```python
from build123d import *
from build123d.topology import SkipClean

# Parameters (mm, degrees)
SKETCH1_R               = 15
SKETCH1_R_2             = 12.5
BOSS_EXTRUDE2_DEPTH     = 2.5
CUT_EXTRUDE2_DEPTH      = 22.360009363
CUT_EXTRUDE2_DEPTH_BACK = 22.360009363
SKETCH3_R               = 0.45
SKETCH4_R               = 1.25
BOSS_EXTRUDE3_DEPTH     = 18
BOSS_EXTRUDE4_START     = -20
SKETCH6_R               = 1.25
BOSS_EXTRUDE4_DEPTH     = 20
SKETCH9_R               = 1.75
BOSS_EXTRUDE5_DEPTH     = 2


with BuildPart() as part:
    # Sketch1 → Boss-Extrude2 (new body)
    with BuildSketch(Plane(origin=(0, 0, 0), x_dir=(1, 0, 0), z_dir=(0, 1, 0))):
        with Locations(Location((0, 0, 0), (0, 0, 270))):
            Circle(SKETCH1_R)
        with Locations(Location((0, 0, 0), (0, 0, 270))):
            Circle(SKETCH1_R_2, mode=Mode.SUBTRACT)
    extrude(amount=BOSS_EXTRUDE2_DEPTH)

    # Sketch3 → Cut-Extrude2 (cut, two sides: drawn at the far end of the back side and taken through both)
    with BuildSketch(Plane.XY.offset(-CUT_EXTRUDE2_DEPTH_BACK)):
        with Locations(Location((0, 1.25, 0), (0, 0, 89.999999951))):
            Circle(SKETCH3_R)
    extrude(amount=CUT_EXTRUDE2_DEPTH + CUT_EXTRUDE2_DEPTH_BACK, mode=Mode.SUBTRACT)

    # Sketch4 → Boss-Extrude3 (add)
    with SkipClean():  # the faces are left unmerged after this step: merging them gives an invalid solid
        with BuildSketch(Plane(origin=(14, 0, 0), x_dir=(0, 0, -1), z_dir=(1, 0, 0))):
            with Locations(Location((0, 1.25, 0), (0, 0, 90))):
                Circle(SKETCH4_R)
        extrude(amount=BOSS_EXTRUDE3_DEPTH)

    # Sketch5 → Revolve1 (revolve)
    with SkipClean():  # the faces are left unmerged after this step: merging them gives an invalid solid
        with BuildSketch(Plane(origin=(32, 0, 0), x_dir=(0, 0, -1), z_dir=(1, 0, 0))):
            with BuildLine():
                Line((0, 2.5), (0, 0))
                ThreePointArc((0, 0), (1.25, 1.25), (0, 2.5))
            make_face()
        revolve(axis=Axis((32, 2.5, 0), (0, -1, 0)))

    # Sketch6 → Boss-Extrude4 (add)
    with BuildSketch(Plane(origin=(-14, 0, 0), x_dir=(0, 0, -1), z_dir=(1, 0, 0)).offset(BOSS_EXTRUDE4_START)):
        with Locations(Location((0, 1.25, 0), (0, 0, 90))):
            Circle(SKETCH6_R)
    extrude(amount=BOSS_EXTRUDE4_DEPTH)

    # Sketch7 → Revolve2 (revolve)
    with BuildSketch(Plane.ZY.offset(34)):
        with BuildLine():
            Line((0, 2.5), (0, 0))
            ThreePointArc((0, 0), (1.25, 1.25), (0, 2.5))
        make_face()
    revolve(axis=Axis((-34, 2.5, 0), (0, -1, 0)))

    # Sketch9 → Boss-Extrude5 (add)
    with BuildSketch(Plane(origin=(24, 0, 0), x_dir=(0, 0, -1), z_dir=(1, 0, 0))):
        with Locations((0, 1.25)):
            Circle(SKETCH9_R)
    extrude(amount=-BOSS_EXTRUDE5_DEPTH)


solid = part.part
```
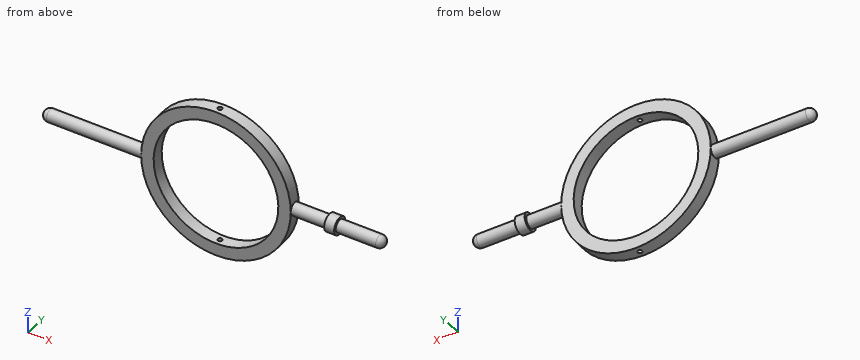
Part model, mm, in its own coordinate system. Round coordinates to 2 decimals unless told otherwise and drop trailing zeros. Loops run counter-clockwise (first coordinate to the right, second up) from the corner with the lowest first, then second, coordinate; pieces in that order, holes last. Notation, with made-up numbers: (-22, -32) -> (-16, -32) arc R26 cw to (-16, -15) -> close; hole circle Ø3 at (32.25, -34.75). An arc over 180 degrees is marked (long way). Use one line per item in the form item = value. Start each with the question number.
Item 1: Band-saw the part on B-B (z = 3). List the corners of the cut face in (x, y), plus the area to 3 significant figures.
Item 2: Band-saw the part on C-C (x = 28). List the corners of the cut face in (y, z).
Item 3: Drop flat-ended pins along their axis: pin 1 Ø1.5 at (y, z) = (0.5, 5.5) entering from -X; pin 2 Ø2 at (x, y) = (-17, 2) entering from +Z; pin 3 Ø1 at (y, z) = (0.5, -0.5) entering from -X. Give the stop position or say it passes through.
Item 4: Band-saw the part on A-A (x = -6.5). List the corners of the cut face in (y, z).
Item 5: Drill centre lines: line 1 along Z through (x, y) = (0, 0.6); line 2 along X through (y, z) = (0.3, -2); line 3 along X through (y, z) = (1.25, 13.55). Where is each one in solid material? Low to high.
Data:
q1.outline = (-14.7, 0) -> (-12.13, 0) -> (-12.13, 2.5) -> (-14.7, 2.5) -> close; (12.13, 0) -> (14.7, 0) -> (14.7, 2.5) -> (12.13, 2.5) -> close
q1.area = 12.8 mm^2
q2.outline = circle Ø2.5 at (1.25, 0)
q3.pin_1 = -14.23
q3.pin_2 = 1.25
q3.pin_3 = -35.18
q4.outline = (0, -13.52) -> (2.5, -13.52) -> (2.5, -10.68) -> (0, -10.68) -> close; (0, 10.68) -> (2.5, 10.68) -> (2.5, 13.52) -> (0, 13.52) -> close
q5.line_1 = -15 to -12.5, 12.5 to 15
q5.line_2 = -14.87 to -12.34, 12.34 to 14.87
q5.line_3 = -6.43 to -0.45, 0.45 to 6.43
